```python
from build123d import *

# Parameters (mm, degrees)
PAD102_DEPTH            = 20
THICKNESS001_T          = -3
POCKET077_DEPTH         = 5
POCKET078_DEPTH         = 5
BODY127_PLACEMENT_ANGLE = 90


with BuildPart() as part:
    # Sketch211 (on XZ_Plane1033 of Origin1405) → Pad102 (new body)
    with BuildSketch(Plane.XZ):
        Polygon((0, 0), (0, 20), (4, 20), (20, 4), (20, 0), align=None)
    extrude(amount=PAD102_DEPTH)

    # Thickness001
    thickness001_openings = [part.faces().sort_by_distance(p)[0] for p in [
        (2, -10, 20),
        (12, -10, 12),
        (20, -10, 2),
    ]]
    offset(amount=THICKNESS001_T, openings=thickness001_openings)

    # Sketch212 (on Face11 of Thickness001) → Pocket077 (cut)
    with BuildSketch(Plane.YZ.offset(3)):
        with BuildLine():
            ThreePointArc((-7, 13), (-10, 16), (-13, 13))
            Line((-13, 13), (-13, 10))
            ThreePointArc((-13, 10), (-10, 7), (-7, 10))
            Line((-7, 13), (-7, 10))
        make_face()
    extrude(amount=-POCKET077_DEPTH, mode=Mode.SUBTRACT)

    # Sketch213 (on Face16 of Pocket077) → Pocket078 (cut)
    with BuildSketch(Plane.XY.offset(3)):
        with BuildLine():
            ThreePointArc((10, -7), (7, -10), (10, -13))
            Line((10, -13), (13, -13))
            ThreePointArc((13, -13), (16, -10), (13, -7))
            Line((10, -7), (13, -7))
        make_face()
    extrude(amount=-POCKET078_DEPTH, mode=Mode.SUBTRACT)


with BuildPart() as part_1:
    # Body127 placement: moved
    add(part.part.moved(Location((-160, 270, -33))).rotate(Axis((-160, 270, -33), (0, 0, 1)), BODY127_PLACEMENT_ANGLE))


solid = part_1.part
```
Could you check a few things on this model? Use its own coordinates, in mm. A direction names the side the tool comes from. Coordinates: 2 decimals unless noted, no trailing zeros. Write each loop counter-clockwise with the first axis right and the second up, starting at its lowest first coordinate (ties: lowest second). Pieces come first, ordered by that corner, then holes. Notation, with made-up numbers: (70.25, 59.25) - (100.25, 59.25) arc R10 cw to (100.25, 71.25) - close; hole circle Ø10 at (-15.5, 78). An arc over 180 degrees is marked (long way). Use a Markdown table: item, result.
Q1. Which directions (+Z, -Z, +X, -X, +Y, -Y) give clear straight access to the entire face, cutting with the end or side of a thin tool? Please do faces 1 (the flat face through (-147, 272, -21)), 2 (the flat face through (-152.4, 270, -25.4)), 3 (the cylindrical face through (-150, 277, -31)), 4 (the flat face through (-157, 280, -23)).
Geometry check:
| item | result |
|---|---|
| face 1 | +Y, -Y |
| face 2 | +Z, -Z, +X, -X, -Y |
| face 3 | +Z, -Z |
| face 4 | +Z, +Y |
Q2. Imagine slicing it at C-C (y = 285). List the corners of the cut face in (x, z) for me, and give its area (3 significant figures).
Geometry check:
| item | result |
|---|---|
| outline | (-160, -33) - (-152.24, -33) - (-152.24, -30) - (-157, -30) - (-157, -24) - (-160, -24) - close; (-147.76, -33) - (-140, -33) - (-140, -24) - (-143, -24) - (-143, -30) - (-147.76, -30) - close |
| area | 82.6 mm2 |
Q3. Imagine slicing it at B-B (z = -22.25). List the corners of the cut face in (x, y) for me.
Geometry check:
| item | result |
|---|---|
| outline | (-160, 270) - (-153, 270) - (-153, 273) - (-157, 273) - (-157, 283.25) - (-160, 283.25) - close; (-147, 270) - (-140, 270) - (-140, 283.25) - (-143, 283.25) - (-143, 273) - (-147, 273) - close |
Q4. Imagine slicing it at A-A (x = -150). List the corners of the cut face in (y, z) for me, and give its area (3 significant figures).
Geometry check:
| item | result |
|---|---|
| outline | (270, -33) - (277, -33) - (277, -30) - (273, -30) - (273, -26) - (270, -26) - close; (270, -17) - (273, -17) - (273, -13) - (270, -13) - close; (286, -33) - (290, -33) - (290, -30) - (286, -30) - close |
| area | 57.0 mm2 |
Q5. Thinking about a two-plate mould opening in Y: for faces 5 (the flat face through (-153, 281, -31)), 6 (the cylindrical face through (-150, 286, -31)), 7 (the flat face through (-153, 272, -21)), 8 (the flat face through (-153.2, 273, -21.6)), which applies, +Y half, -Y half, draft (parallel to the pull), parting line (faces both ways), or undercut?
Geometry check:
| item | result |
|---|---|
| face 5 | undercut |
| face 6 | undercut |
| face 7 | draft |
| face 8 | +Y half |
Q6. I'm going to push flat-ended pins straight in: pin 1 Ø5 at (y, z) = (283.5, -21) entering from -X; pin 2 Ø6 at (x, y) = (-144.5, 279) entering from +Z; pin 3 Ø5 at (x, y) = (-149.5, 283.5) entering from +Z. Where does each tip first touch, or does it pass through?
Geometry check:
| item | result |
|---|---|
| pin 1 | stops at x = -160 |
| pin 2 | stops at z = -15.4 |
| pin 3 | stops at z = -30 |
Q7. Imagine slicing it at D-D (z = -29.5). List the corners of the cut face in (x, y) for me.
Geometry check:
| item | result |
|---|---|
| outline | (-160, 270) - (-140, 270) - (-140, 290) - (-143, 290) - (-143, 273) - (-157, 273) - (-157, 290) - (-160, 290) - close |
Q8. Please list where these lines run through material, in increasing order: L1, parallel to X at y = 273.5, z = -20; L2, parallel to X at y = 272, z = -21.75; L3, parallel to Y at x = -148.75, z = -29.
Geometry check:
| item | result |
|---|---|
| L1 | x = -160 to -157, -143 to -140 |
| L2 | x = -160 to -153, -147 to -140 |
| L3 | y = 270 to 273 |
